Verification items for the finished model (mm, model axes). A direction names the side the tool comes from. Give positions to 0.01 mm unless a question says otherwise; leave off trailing zeros. Order: outer loops, then holes, each group sorted by start corner. A loop starts at its lowest first (then second) coordinate and runs counter-clockwise, first axis right, second up. Notation, with made-up numbers: (-29.5, -8) - (0.5, -8) arc R20 cw to (0.5, 30) - close; hole circle Ø2 at (17.25, -33.5). An arc over 180 degrees is marked (long way). Answer as a JSON object with one key per item and string values.
Autodesk Fusion 360 part; units mm, degrees
sketch "Sketch1" plane through (0, 0, 0) normal (0, 0, 1) x (1, 0, 0)
  circle A0 centre (0, 0) radius 30
  dimension "d1" = 60
extrude "Extrude1" add sketch "Sketch1" along normal blind 25
sketch "Sketch2" plane through (0, 0, 25) normal (0, 0, 1) x (-1, 0, 0)
  circle A0 centre (0, 0) radius 30
  circle A1 centre (0, 0) radius 10
  dimension "d4" = 20
extrude "Extrude2" add sketch "Sketch2" along normal blind 25 contours A1
mirror "Mirror1" about plane through (0, 0, 0) normal (0, 0, 1) of bodies 1 merged
(1) Section check D-D (x = 24.5). Record the cut outline in (y, z), then the cut area to 3 significant figures.
Computed values:
{"outline": "(-17.31, -25) - (17.31, -25) - (17.31, 25) - (-17.31, 25) - close", "area": "1,730 mm²"}
(2) Section check A-A (x = 0). Record the cut outline in (y, z).
Computed values:
{"outline": "(-30, -25) - (-10, -25) - (-10, -50) - (10, -50) - (10, -25) - (30, -25) - (30, 25) - (10, 25) - (10, 50) - (-10, 50) - (-10, 25) - (-30, 25) - close"}
(3) Gauge pin test, flat ends, axial feed: pin 1 Ø6 at (x, z) = (-7.5, 10.5) entering from +Y; pin 2 Ø2 at (y, z) = (-11.5, 7.5) entering from -X; pin 3 Ø6 at (y, z) = (11.5, -11.5) entering from +X; pin 4 Ø18 at (x, y) = (-11, 8) entering from -Z. Record the tip position at first contact, or that the pin passes through.
Computed values:
{"pin 1": "stops at y = 29.66", "pin 2": "stops at x = -28.1", "pin 3": "stops at x = 28.77", "pin 4": "stops at z = -50"}
(4) Access from +Z, -Z, +X, -X, +Y, -Y to the whole of each face (thin tool, end or side, straight path). Record for faces 1 (the cylindrical face through (2.17, 9.76, -37.33)), 2 (the flat face through (13, 0, 25)), 3 (the cylindrical face through (-29.97, -1.32, -0.35)).
Computed values:
{"face 1": "-Z", "face 2": "+Z", "face 3": "+Z, -Z"}
(5) Material ranges on line 1 along Z through (x, y) = (15, -6.5); line 2 along Y through (x, z) = (1, 13.5); line 3 along X through (y, z) = (-17, 7.5), recorded low to high. Write a range as [from, to].
Computed values:
{"line 1": "z = [-25, 25]", "line 2": "y = [-29.98, 29.98]", "line 3": "x = [-24.72, 24.72]"}
(6) Section check C-C (z = -15.5). Record the cut outline in (x, y).
Computed values:
{"outline": "circle Ø60 at (0, 0)"}
